For this review, take the finished solid that the model builds, in its own axes (mm). A direction names the side the tool comes from. Coordinates: 2 decimals unless noted, no trailing zeros. Write each loop counter-clockwise with the first axis right and the second up, starting at its lowest first coordinate (ties: lowest second). Pieces come first, ordered by that corner, then holes. Notation, with made-up numbers: (-6.75, 19.25) -> (37.25, 19.25) arc R26 cw to (37.25, 34.25) -> close; hole circle Ø11 at (-12.5, 59.5). An arc over 180 degrees is marked (long way). Put each result on its own line as item: value. Start each with the question number.
Item 1: Consider section A-A on y = -17. Give the boundary of the cut face in (x, z), and give its area (3 significant figures).
Item 2: Consider section D-D on x = 26.5. Give the boundary of the cut face in (y, z).
Item 3: Insertion check: P1, Ø8, axis at x = 5, z = -19.5, coming from the -Y side; P2, Ø1.5, axis at x = 12.5, y = -13, coming from the +Z side; P3, Ø6.5, axis at x = -1, y = -16.5, coming from the +Z side; P4, Ø18.5, axis at y = -18.5, z = -11.5, coming from the -X side. Each pin has a flat end and moves straight along its axis. Give the tip position at first contact, or say it passes through.
Item 4: To check wall thickness, follow L1, parallel to Y at x = -3.5, z = -13.5; L2, parallel to Z at x = -7.5, y = -13; L3, parallel to X at y = -25, z = 21. State the ranges of each line that lie inside material, in increasing order.
Item 5: Consider section B-B on x = 18. Give the boundary of the cut face in (y, z).
Item 6: The part is to be moulded in two halves that separate along Y. For faces 1 (the flat face through (-15.901, -9, -5)), 2 (the flat face through (14, 26, -7)), 3 (the flat face through (-14, -55, 2)), 4 (the flat face through (7, 4, -26)), say which applies: +Y half, -Y half, draft (parallel to the pull), parting line (faces both ways), or undercut.
Item 7: Consider section C-C on z = 5. Give the boundary of the cut face in (x, y), and give its area (3 significant figures).
Item 8: For faces 5 (the flat face through (-29, -9, 18.49)), 6 (the flat face through (7, -30, -26)), 7 (the flat face through (-1, -13, 2.49)), list the 3-axis set-ups (+Z, -Z, +X, -X, +Y, -Y) from which the entire face can be reached by the end or side of a thin tool; tool diameter is ignored.
```python
from build123d import *

# Parameters (mm, degrees)
F1_DEPTH  = 55
F2_W      = 34
F2_H      = 46
F3_DEPTH  = 28
F5_DEPTH  = 34
F6_R      = 12.5
F8_DEPTH  = 100
F10_DEPTH = 17
F11_W     = 12
F11_H     = 74
F12_DEPTH = 24
F14_DEPTH = 12
F15_DEPTH = 12
F16_R     = 12
F17_DEPTH = 25


# Not quite as in the source:
# - a feature of the source that left no trace in its solid (it failed there, or was rolled back) is left out


with BuildPart() as f1:
    # F0 (on Front) → F1 (new body, symmetric)
    with BuildSketch(Plane.XZ):
        Polygon((-3.9005428076, 30.4901414615), (-40.9005428076, 30.4901414615), (-40.9005428076, 18.4901414615), (-15.9005428076, 18.4901414615), (-15.9005428076, -43.5098585385), (-3.9005428076, -43.5098585385), align=None)
    extrude(amount=F1_DEPTH, both=True)

    # F2 (on face) → F3 (join)
    with BuildSketch(Plane.YZ.offset(-3.9005428076)):
        with Locations((-13, -20.5098585385)):
            Rectangle(F2_W, F2_H)
    extrude(amount=F3_DEPTH)

    # F4 (on face) → F5 (cut)
    with BuildSketch(Plane.XZ.offset(30)):
        Polygon((24.0994571924, 2.4901414615), (2.0994571924, 2.4901414615), (24.0994571924, -37.5098585385), align=None)
    extrude(amount=-F5_DEPTH, mode=Mode.SUBTRACT)

    # F6 (on face) → F8 (cut)
    with BuildSketch(Plane(origin=(-15.9005428076, 0, 0), x_dir=(0, -1, 0), z_dir=(-1, 0, 0))):
        with Locations((13, -20.5098585385)):
            Circle(F6_R)
    extrude(amount=-F8_DEPTH, mode=Mode.SUBTRACT)

    # F10 (cut): a face of the model
    f10_faces = [f1.faces().sort_by_distance(p)[0] for p in [
        (-14.5722599793, 55, 1.3184242898),
    ]]
    extrude(f10_faces, amount=-F10_DEPTH, mode=Mode.SUBTRACT)

    # F11 (on face) → F12 (join)
    with BuildSketch(Plane.YZ.offset(-3.9005428076)):
        with Locations((32, -6.5098585385)):
            Rectangle(F11_W, F11_H)
    extrude(amount=F12_DEPTH)

    # F13 (on face) → F14 (cut)
    with BuildSketch(Plane(origin=(0, 38, 0), x_dir=(-1, 0, 0), z_dir=(0, 1, 0))):
        with BuildLine():
            ThreePointArc((-20.0994571924, -17.5098585385), (-28.0551210727, -16.1529018901), (-35.1111607034, -12.2354762238))
            Line((-35.1111607034, -12.2354762238), (-20.0994571924, -24.2698585385))
            Line((-20.0994571924, -24.2698585385), (-20.0994571924, -17.5098585385))
        make_face()
        Polygon((3.9005428076, -43.5098585385), (-20.0994571924, -24.2698585385), (-20.0994571924, -43.5098585385), align=None)
    extrude(amount=-F14_DEPTH, mode=Mode.SUBTRACT)

    # F13 (on face) → F15 (join)
    with BuildSketch(Plane(origin=(0, 38, 0), x_dir=(-1, 0, 0), z_dir=(0, 1, 0))):
        with BuildLine():
            ThreePointArc((-35.1111607034, -12.2354762238), (-9.7139115703, -15.1464119177), (3.9005428076, 6.4901414615))
            ThreePointArc((3.9005428076, 6.4901414615), (-3.1288944439, 23.46070421), (-20.0994571924, 30.4901414615))
            ThreePointArc((-20.0994571924, 30.4901414615), (-42.742500544, 14.4458053418), (-35.1111607034, -12.2354762238))
        make_face()
        with BuildLine():
            ThreePointArc((-20.0994571924, -17.5098585385), (-28.0551210727, -16.1529018901), (-35.1111607034, -12.2354762238))
            Line((-35.1111607034, -12.2354762238), (-20.0994571924, -24.2698585385))
            Line((-20.0994571924, -24.2698585385), (-20.0994571924, -17.5098585385))
        make_face()
    extrude(amount=-F15_DEPTH)

    # F16 (on face) → F17 (cut)
    with BuildSketch(Plane(origin=(0, 38, 0), x_dir=(-1, 0, 0), z_dir=(0, 1, 0))):
        with Locations((-20.0994571924, 6.4901414615)):
            Circle(F16_R)
    extrude(amount=-F17_DEPTH, mode=Mode.SUBTRACT)


solid = f1.part
```
Return value:
1. outline: (-40.9, 18.49) -> (-15.9, 18.49) -> (-15.9, -8.67) -> (8.24, -8.67) -> (2.1, 2.49) -> (-3.9, 2.49) -> (-3.9, 30.49) -> (-40.9, 30.49) -> close; (-15.9, -43.51) -> (24.1, -43.51) -> (24.1, -37.51) -> (21.26, -32.35) -> (-15.9, -32.35) -> close
1. area: 1,310 mm^2
2. outline: (26, -19.14) -> (38, -19.14) -> (38, -3.66) -> (26, -3.66) -> close; (26, 16.64) -> (38, 16.64) -> (38, 29.62) -> (26, 29.62) -> close
3. P1: y = -30
3. P2: z = -32.99
3. P3: z = 30.49
3. P4: x = -15.9
4. L1: -30 to -23.35, -2.65 to 4, 26 to 38
4. L2: -43.51 to -33.01, -8.01 to 30.49
4. L3: -40.9 to -3.9
5. outline: (-30, -43.51) -> (4, -43.51) -> (4, -26.42) -> (-1.99, -26.42) arc R12.5 cw to (-24.01, -26.42) -> (-30, -26.42) -> close; (26, -25.95) -> (38, -25.95) -> (38, -5.32) -> (26, -5.32) -> close; (26, 18.31) -> (38, 18.31) -> (38, 30.49) -> (26, 30.49) -> close
6. face 1: draft
6. face 2: undercut
6. face 3: -Y half
6. face 4: undercut
7. outline: (-15.9, -55) -> (-3.9, -55) -> (-3.9, 26) -> (8.19, 26) -> (8.19, 38) -> (-15.9, 38) -> close; (32.01, 26) -> (44.05, 26) -> (44.05, 38) -> (32.01, 38) -> close
7. area: 1,410 mm^2
8. face 5: -Z, -X, +Y, -Y
8. face 6: +Z, -Z, +X, -Y
8. face 7: +Z, +X, -Y
